Autodesk Inventor part; units mm, degrees
ref_plane "YZ Plane" through (0, 0, 0) normal (1, 0, 0) x (0, 1, 0)
ref_plane "XZ Plane" through (0, 0, 0) normal (0, 1, 0) x (-1, 0, 0)
ref_plane "XY Plane" through (0, 0, 0) normal (0, 0, 1) x (1, 0, 0)
sketch "スケッチ1" plane through (0, 0, 0) normal (0, 0, 1) x (1, 0, 0)
  line L0 (0, 0) -> (25, 0)
  line L1 (25, 0) -> (25, 4)
  line L2 (25, 4) -> (0, 4)
  line L3 (0, 4) -> (0, 0)
  dimension "d0" = 4
  dimension "d1" = 25
extrude "押し出し1" add sketch "スケッチ1" along normal blind 18.9
sketch "スケッチ2" plane through (0, 4, 0) normal (0, 1, 0) x (1, 0, 0)
  line L0 (0, 0) -> (0, -18.9)
  line L1 (25, 0) -> (25, -18.9)
  line L2 (0, 0) -> (25, 0)
  line L3 (25, 0) -> (25, -8)
  line L4 (25, -8) -> (0, -8)
  line L5 (0, -8) -> (0, 0)
  point P0 (0, -8)
  dimension "d4" = 8
extrude "押し出し2" add sketch "スケッチ2" along normal blind 30
sketch "スケッチ3" plane through (0, 4, 18.9) normal (0, 1, 0) x (1, 0, 0)
  line L0 (0, 10.9) -> (25, 10.9)
  line L1 (25, 10.9) -> (25, 0)
  point P0 (0, 18.9)
  point P1 (5, 4.5)
  point P2 (20, 4.5)
  dimension "d7" = 15
  dimension "d8" = 6.4
  dimension "d9" = 6.4
  dimension "d10" = 5
hole "穴1" at (5, 4, 14.4) at (20, 4, 14.4) direction (0, -1, 0) diameter 5 end through all
sketch "スケッチ4" plane through (0, 4, 8) normal (0, 0, 1) x (1, 0, 0)
  line L0 (25, 0) -> (0, 0)
  line L1 (0, 0) -> (0, 30)
  point P0 (0, -4)
  point P1 (5, 7)
  point P2 (20, 7)
  dimension "d18" = 7
  dimension "d19" = 7
  dimension "d20" = 15
  dimension "d21" = 5
hole "穴2" at (5, 11, 8) at (20, 11, 8) direction (0, 0, -1) diameter 5 end through all
sketch "スケッチ7" plane through (0, 4, 18.9) normal (0, 1, 0) x (1, 0, 0)
  line L0 (25, 10.9) -> (0, 10.9)
  line L1 (25, 0) -> (0, 0)
  line L2 (10, 10.9) -> (15, 10.9)
  line L3 (15, 10.9) -> (15, 0)
  line L4 (15, 0) -> (10, 0)
  line L5 (10, 0) -> (10, 10.9)
  line L6 (25, 10.9) -> (25, 0)
  point P0 (0, 18.9)
  point P1 (10, 0)
  point P2 (15, 10.9)
  dimension "d36" = 5
  dimension "d37" = 10
extrude "押し出し5" add sketch "スケッチ7" along normal blind 15 contours L3 L1 L5 L0
sketch "スケッチ8" plane through (10, 4, 8) normal (-1, 0, 0) x (0, 0, 1)
  line L0 (10.9, 0) -> (0, 0)
  line L1 (10.9, 0) -> (10.9, 15)
  line L2 (0, 15) -> (10.9, 15)
  line L3 (0, 0) -> (0, 15)
  line L4 (10.9, 0) -> (0, 15)
  point P0 (-8, -4)
extrude "押し出し6" cut sketch "スケッチ8" against normal blind 15 contours L4 L2 L1
fillet "フィレット1" radius 2 7 edges at (0, 34, 4) (25, 34, 4) (25, 2, 18.9) (0, 2, 18.9) (20, 4, 8) (5, 4, 8) (12.5, 4, 18.9)
sketch "スケッチ9" plane through (0, 0, 0) normal (0, 0, -1) x (-1, 0, 0)
  line L0 (-37.1274, 50.0053) -> (12.2795, 50.0053)
  line L1 (12.2795, 50.0053) -> (12.2795, -2.3527)
  line L2 (12.2795, -2.3527) -> (-37.1274, -2.3527)
  line L3 (-37.1274, -2.3527) -> (-37.1274, 50.0053)
  point P0 (0, 0)
extrude "押し出し7" cut sketch "スケッチ9" against normal blind 4
properties part number "BP_L"
Work out the finished part from the listing and answer in its coordinate system (mm). A direction names the side the tool comes from. Round coordinates to 2 decimals unless told otherwise and drop trailing zeros. Order: outer loops, then holes, each group sorted by start corner. A loop starts at its lowest first (then second) coordinate and runs counter-clockwise, first axis right, second up.
Q1. A cutting plane is placed at C-C, the plane z = 16. Determine the outline of the cut face in (x, y).
Solution:
outline: (0, 0) - (3.08, 0) - (3.08, 4) - (0, 4) - close; (6.92, 0) - (18.08, 0) - (18.08, 4) - (15, 4) - (15, 7.99) - (10, 7.99) - (10, 4) - (6.92, 4) - close; (21.92, 0) - (25, 0) - (25, 4) - (21.92, 4) - close
Q2. Given pin 1 Ø2.5 at (x, z) = (7.5, 14) entering from +Y; pin 2 Ø2 at (x, z) = (15.5, 15.5) entering from +Y; pin 3 Ø3 at (x, z) = (12.5, 12.5) entering from +Y, each flat-ended and moving along its own axis, determine where each tip first touches the part or whether it passes through.
Solution:
pin 1: stops at y = 4
pin 2: stops at y = 9.87
pin 3: stops at y = 14.87
Q3. A cutting plane is placed at B-B, the plane x = 5. Determine the outline of the cut face in (y, z).
Solution:
outline: (0, 4) - (8.5, 4) - (8.5, 8) - (6, 8) arc R2 cw to (4, 10) - (4, 11.9) - (0, 11.9) - close; (0, 16.9) - (4, 16.9) - (4, 18.9) - (0, 18.9) - close; (13.5, 4) - (34, 4) - (34, 8) - (13.5, 8) - close
Q4. Find the intervals of material crossed by line 1 along Z through (x, y) = (5, 2.8); line 2 along Y through (x, z) = (20, 6.6); line 3 along Y through (x, z) = (9, 18.25), in increasing order.
Solution:
line 1: z = 4 to 11.9, 16.9 to 18.9
line 2: y = 0 to 8.5, 13.5 to 34
line 3: y = 0 to 4
Q5. A tool of negligible diameter and unlimited length cuts with its end or side. For faces 1 (the flat face through (13, 20, 8)), 2 (the flat face through (15, 10, 12)), from which of +Z, -Z, +X, -X, +Y, -Y can it reach the whole face along a straight path? Write none if from no direction.
Solution:
face 1: +Z, +Y
face 2: +Z, +X, +Y
Q6. A cutting plane is placed at A-A, the plane y = 13. Determine the outline of the cut face in (x, z).
Solution:
outline: (0, 4) - (3.5, 4) - (3.5, 8) - (0, 8) - close; (6.5, 4) - (18.5, 4) - (18.5, 8) - (15, 8) - (15, 12.36) - (10, 12.36) - (10, 8) - (6.5, 8) - close; (21.5, 4) - (25, 4) - (25, 8) - (21.5, 8) - close
Q7. A cutting plane is placed at D-D, the plane x = 13.25. Determine the outline of the cut face in (y, z).
Solution:
outline: (0, 4) - (34, 4) - (34, 8) - (19, 8) - (4.53, 18.52) arc R2 ccw to (3.35, 18.9) - (0, 18.9) - close
Q8. The mould has two halves that part along Y. Classify faces 3 (the cylindrical face through (24.4, 2.03, 18.33)), 4 (the cylindrical face through (19.93, 4.6, 8.57)), 5 (the flat face through (12, 0, 11)), 6 (the cylindrical face through (17.52, 11.33, 5.97)): pulls with the +Y half, pulls with the -Y half, needs draft (parallel to the pull), parting line crosses it, or undercut.
Solution:
face 3: needs draft
face 4: pulls with the +Y half
face 5: pulls with the -Y half
face 6: undercut
